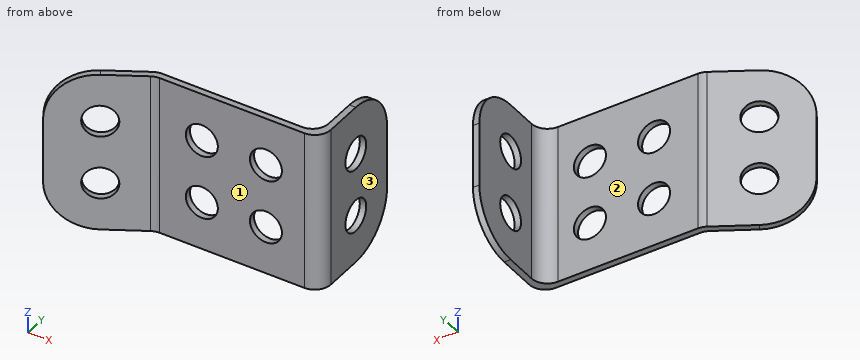
from build123d import *

# Parameters (mm, degrees)
EXTRUDE_THIN1_DEPTH  = 50
FILLET1_R            = 15
CUT_EXTRUDE1_REACH   = 79.453
SKETCH2_R            = 5
LPATTERN1_COUNT      = 2
LPATTERN1_PITCH      = 20
LPATTERN1_COUNT_DIR2 = 2
LPATTERN1_PITCH_DIR2 = 20
CUT_EXTRUDE2_REACH   = 74.528
SKETCH3_R            = 5
SKETCH4_R            = 5
CUT_EXTRUDE3_DEPTH   = 96.776177682
LPATTERN2_COUNT      = 2
LPATTERN2_PITCH      = 20
FILLET2_R            = 5


with BuildPart() as part:
    # Sketch1 → Extrude-Thin1 (new body)
    with BuildSketch(Plane.XY):
        Polygon((25, 30), (25, 0), (-25, 0), (-50.980762114, -15), (-49.980762114, -16.732050808), (-24.464101615, -2), (27, -2), (27, 30), align=None)
    extrude(amount=EXTRUDE_THIN1_DEPTH)

    # Fillet1
    fillet1_edges = [part.edges().sort_by_distance(p)[0] for p in [
        (-50.480762114, -15.866025404, 50),
        (-50.480762114, -15.866025404, 0),
        (26, 30, 50),
        (26, 30, 0),
    ]]
    fillet(fillet1_edges, radius=FILLET1_R)

    # Sketch2 → Cut-Extrude1 (cut, up to next)
    with BuildSketch(Plane(origin=(0, 0, 0), x_dir=(1, 0, 0), z_dir=(0, 1, 0)), mode=Mode.PRIVATE) as cut_extrude1_sk1:
        with Locations(Location((-10, -15, 0), (0, 0, 180))):
            Circle(SKETCH2_R)
    cut_extrude1_tool1 = extrude(cut_extrude1_sk1.sketch, amount=-CUT_EXTRUDE1_REACH, mode=Mode.PRIVATE) & part.part
    cut_extrude1 = cut_extrude1_tool1.solids().sort_by_distance((-10, 0, 15))[0]
    add(cut_extrude1, mode=Mode.SUBTRACT)

    # LPattern1: Cut-Extrude1 2 × 2
    with Locations(*[(j * LPATTERN1_PITCH_DIR2, 0, i * LPATTERN1_PITCH) for i in range(LPATTERN1_COUNT) for j in range(LPATTERN1_COUNT_DIR2) if (i, j) != (0, 0)]):
        add(cut_extrude1, mode=Mode.SUBTRACT)

    # Sketch3 → Cut-Extrude2 (cut, up to next)
    with BuildSketch(Plane(origin=(-6.25, 10.825317547, 0), x_dir=(0.8660254037844379, 0.5000000000000013, 0), z_dir=(-0.5000000000000013, 0.8660254037844379, 0)), mode=Mode.PRIVATE) as cut_extrude2_sk1:
        with Locations(Location((-36.650635095, -15, 0), (0, 0, 180))):
            Circle(SKETCH3_R)
    cut_extrude2_tool1 = extrude(cut_extrude2_sk1.sketch, amount=-CUT_EXTRUDE2_REACH, mode=Mode.PRIVATE) & part.part
    # Sketch3 → Cut-Extrude2 (cut, up to next)
    with BuildSketch(Plane(origin=(-6.25, 10.825317547, 0), x_dir=(0.8660254037844379, 0.5000000000000013, 0), z_dir=(-0.5000000000000013, 0.8660254037844379, 0)), mode=Mode.PRIVATE) as cut_extrude2_sk2:
        with Locations(Location((-36.650635095, -35, 0), (0, 0, 180))):
            Circle(SKETCH3_R)
    cut_extrude2_tool2 = extrude(cut_extrude2_sk2.sketch, amount=-CUT_EXTRUDE2_REACH, mode=Mode.PRIVATE) & part.part
    add(cut_extrude2_tool1.solids().sort_by_distance((-37.990381, -7.5, 15))[0], mode=Mode.SUBTRACT)
    add(cut_extrude2_tool2.solids().sort_by_distance((-37.990381, -7.5, 35))[0], mode=Mode.SUBTRACT)

    # Sketch4 → Cut-Extrude3 (cut, through all)
    with BuildSketch(Plane.ZY.offset(-25)):
        with Locations((15, 15)):
            Circle(SKETCH4_R)
    cut_extrude3 = extrude(amount=-CUT_EXTRUDE3_DEPTH, mode=Mode.SUBTRACT)

    # LPattern2: Cut-Extrude3 ×2
    with Locations(*[(0, 0, i * LPATTERN2_PITCH) for i in range(1, LPATTERN2_COUNT)]):
        add(cut_extrude3, mode=Mode.SUBTRACT)

    # Fillet2
    fillet2_edges = [part.edges().sort_by_distance(p)[0] for p in [
        (27, -2, 25),
        (-24.464101615, -2, 25),
        (-25, 0, 25),
        (25, 0, 25),
    ]]
    fillet(fillet2_edges, radius=FILLET2_R)


solid = part.part
Could you check a few things on this model? Use its own coordinates, in mm. Face numbers are marked on the shaded views. A direction names the side the tool comes from. Round coordinates to 2 decimals unless told otherwise and drop trailing zeros. Loops run counter-clockwise (first coordinate to the right, second up) from the corner with the lowest first, then second, coordinate; pieces in that order, holes last. Notation, with made-up numbers: (49.25, 71.5) - (59.25, 71.5) arc R11 cw to (59.25, 79.5) - close; hole circle Ø11 at (79.25, 87). An arc over 180 degrees is marked (long way). Write item = value, one per line.
1) Imagine slicing it at A-A (x = -10). Please give me the cut outline in (y, z).
Computed:
outline = (-2, 0) - (0, 0) - (0, 10) - (-2, 10) - close; (-2, 20) - (0, 20) - (0, 30) - (-2, 30) - close; (-2, 40) - (0, 40) - (0, 50) - (-2, 50) - close
2) Imagine slicing it at B-B (z = 14). Please give me the cut outline in (x, y).
Computed:
outline = (-50.95, -14.98) - (-49.95, -16.72) - (-41.23, -11.68) - (-42.23, -9.95) - close; (-33.75, -5.05) - (-32.75, -6.78) - (-25.62, -2.67) arc R5 cw to (-23.12, -2) - (-14.9, -2) - (-14.9, 0) - (-23.66, 0) arc R5 ccw to (-26.16, -0.67) - close; (-5.1, -2) - (5.1, -2) - (5.1, 0) - (-5.1, 0) - close; (14.9, -2) - (22, -2) arc R5 ccw to (27, 3) - (27, 10.1) - (25, 10.1) - (25, 5) arc R5 cw to (20, 0) - (14.9, 0) - close; (25, 19.9) - (27, 19.9) - (27, 29.97) - (25, 29.97) - close
3) Imagine slicing it at C-C (x = 8). Please give me the cut outline in (y, z).
Computed:
outline = (-2, 0) - (0, 0) - (0, 10.42) - (-2, 10.42) - close; (-2, 19.58) - (0, 19.58) - (0, 30.42) - (-2, 30.42) - close; (-2, 39.58) - (0, 39.58) - (0, 50) - (-2, 50) - close
4) I'm going to push flat-ended pins straight in: P1, Ø9, axis at x = 10, z = 35, coming from the -Y side; P2, Ø13, axis at x = -5.5, z = 30, coming from the +Y side; P3, Ø11.5, axis at y = 15, z = 15, coming from the -X side; P4, Ø16, axis at x = 10, z = 15, coming from the -Y side. Where does each tip first touch, or does it pass through?
Computed:
P1 = through
P2 = 0
P3 = 25
P4 = -2
5) On a 3-axis mill with a long thin cutter (end or side, diameter ignored), from which of +Z, -Z, +X, -X, +Y, -Y can I reach the whole of each face in a straight line? I mean the marked faces 1, 2 and 3. Say none if no direction works.
Computed:
face_1 = +Z, -Z, +X, -Y
face_2 = +Z, -Z, -X, +Y
face_3 = +Z, -Z, +X, +Y, -Y
6) I need wall thicknesses on line 1 along Z through (x, y) = (10, -1.05); line 2 along X through (y, z) = (-1, 31.5); line 3 along Z through (x, y) = (-36, -8.5). Which ranges of each line are inside material? Lowest first, please. Write a range as from..to.
Computed:
line_1 = 0..10, 20..30, 40..50
line_2 = -26.73..-13.57, -6.43..6.43, 13.57..25
line_3 = 0..10.15, 19.85..30.15, 39.85..50
7) Imagine slicing it at D-D (z = 42). Please give me the cut outline in (x, y).
Computed:
outline = (-49.48, -14.13) - (-48.48, -15.87) - (-25.62, -2.67) arc R5 cw to (-23.12, -2) - (22, -2) arc R5 ccw to (27, 3) - (27, 28.27) - (25, 28.27) - (25, 5) arc R5 cw to (20, 0) - (-23.66, 0) arc R5 ccw to (-26.16, -0.67) - close
